Can you work these out from the drawing? Everything is in mm from the part's minimum corner. A direction names the side the tool comes from. Coordinates: 2 decimals unless noted, no trailing zeros. Write each loop counter-clockwise with the first axis right and the second up, starting at its lowest first coordinate (ties: lowest second). Pieces come first, ordered by that corner, then holes. Notation, with made-up numbers: (41, 87) -> (80, 87) arc R16 ccw to (80, 100) -> close; hole circle Ø11 at (31.25, 51). An arc over 180 degrees is marked (long way). Use a Markdown table: item, result. Add a question column.
Item 1: Imagine slicing it at C-C, the plane y = 228.6. Write out the boundary of the cut face in (x, z) (1 decimal).
Item 2: If I drill on line 1 along X through (y, z) = (268.5, 26) (1 decimal); line 2 along X through (y, z) = (228.6, 24.5) (1 decimal); line 3 along Y through (x, z) = (187, 19) (1 decimal), over which ranges is the centre line in solid material (lowest first)? Write a range as from..to.
Item 3: Will these pins go through, and if not, where does the flat tip stop? pin 1 Ø5 at (x, z) = (486, 2) entering from +Y (1 decimal); pin 2 Ø1.5 at (x, z) = (361.5, 21.5) entering from +Y (1 decimal).
Item 4: On a 3-axis mill with a long thin cutter (end or side, diameter ignored), from which of +Z, -Z, +X, -X, +Y, -Y can I reach the whole of each face in a straight line? I mean the marked faces 1 and 2. Say none if no direction works.
Item 5: Imagine slicing it at B-B, the plane z = 31. Write out the boundary of the cut face in (x, y) (1 decimal), and give its area (3 significant figures).
Item 6: Imagine slicing it at A-A, the plane y = 362. Write out the boundary of the cut face in (x, z) (1 decimal).
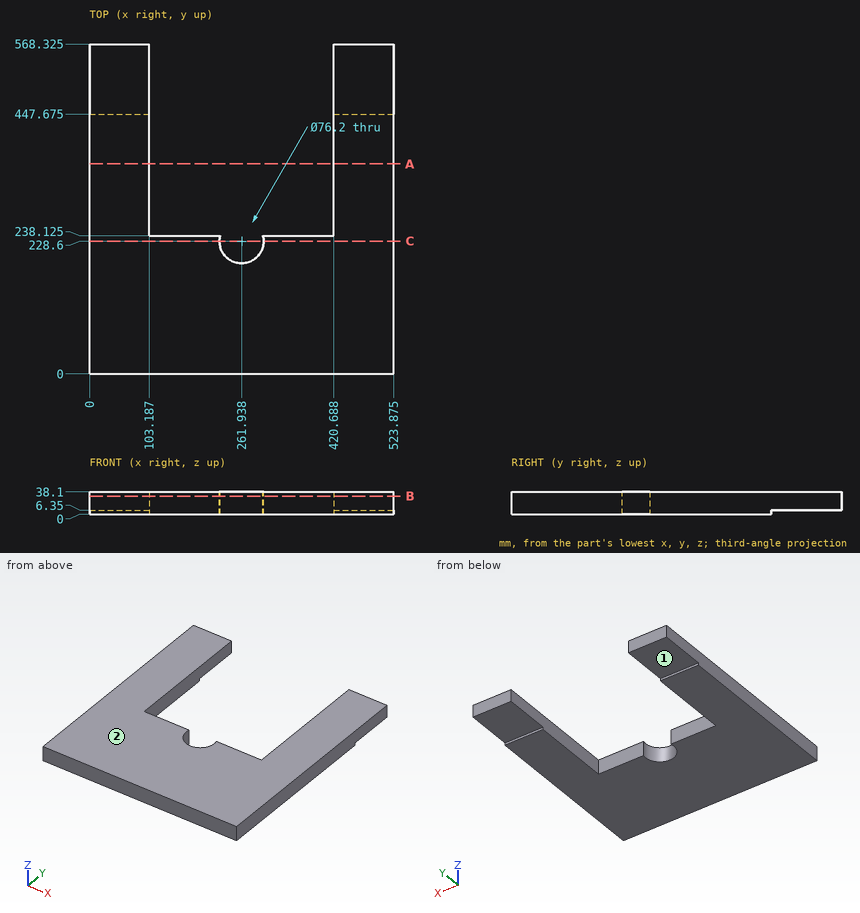
Ans:
| question | item | result |
|---|---|---|
| 1 | outline | (0, 0) -> (223.8, 0) -> (223.8, 38.1) -> (0, 38.1) -> close; (300, 0) -> (523.9, 0) -> (523.9, 38.1) -> (300, 38.1) -> close |
| 2 | line 1 | x = 0..103.2, 420.7..523.9 |
| 2 | line 2 | x = 0..223.8, 300..523.9 |
| 2 | line 3 | y = 0..238.1 |
| 3 | pin 1 | stops at y = 447.7 |
| 3 | pin 2 | stops at y = 238.1 |
| 4 | face 1 | -Z, +X, -X, +Y |
| 4 | face 2 | +Z, +X, -X, +Y, -Y |
| 5 | outline | (0, 0) -> (523.9, 0) -> (523.9, 568.3) -> (420.7, 568.3) -> (420.7, 238.1) -> (298.8, 238.1) arc R38.1 cw (long way) to (225, 238.1) -> (103.2, 238.1) -> (103.2, 568.3) -> (0, 568.3) -> close |
| 5 | area | 190,000 mm^2 |
| 6 | outline | (0, 0) -> (103.2, 0) -> (103.2, 38.1) -> (0, 38.1) -> close; (420.7, 0) -> (523.9, 0) -> (523.9, 38.1) -> (420.7, 38.1) -> close |
